```python
from build123d import *

# Parameters (mm, degrees)
BOSS_EXTRUDE1_DEPTH      = 1.7
BOSS_EXTRUDE1_DEPTH_BACK = 1.7
SKETCH1_R                = 2.7
SKETCH1_R_2              = 1.5
SKETCH1_R_3              = 3.5


with BuildPart() as part:
    # Sketch1 → Boss-Extrude1 (new, two sides: drawn at the far end of the back side and taken through both)
    # profile 1 of 3: a face of its own
    with BuildSketch(Plane(origin=(0, 0, 0), x_dir=(0, 0, -1), z_dir=(1, 0, 0)).offset(-BOSS_EXTRUDE1_DEPTH_BACK)):
        with BuildLine():
            Line((43.152237127, 13.072535054), (4.028300378, -1.651140858))
            ThreePointArc((4.028300378, -1.651140858), (6.515897328, -1.95802161), (7.67928888, -4.178119463))
            ThreePointArc((7.67928888, -4.178119463), (7.169578833, -5.756925949), (5.832896346, -6.739633526))
            Line((5.832896346, -6.739633526), (45.491528196, 6.476340855))
            ThreePointArc((45.491528196, 6.476340855), (41.086299002, 8.626962345), (43.152237127, 13.072535054))
        make_face()
    # profile 2 of 3: a face of its own
    with BuildSketch(Plane(origin=(0, 0, 0), x_dir=(0, 0, -1), z_dir=(1, 0, 0)).offset(-BOSS_EXTRUDE1_DEPTH_BACK)):
        with Locations((4.97928888, -4.178119463)):
            Circle(SKETCH1_R)
        with Locations((4.97928888, -4.178119463)):
            Circle(SKETCH1_R_2, mode=Mode.SUBTRACT)
    # profile 3 of 3: a face of its own
    with BuildSketch(Plane(origin=(0, 0, 0), x_dir=(0, 0, -1), z_dir=(1, 0, 0)).offset(-BOSS_EXTRUDE1_DEPTH_BACK)):
        with Locations((44.385, 9.796822048)):
            Circle(SKETCH1_R_3)
        with Locations((44.385, 9.796822048)):
            Circle(SKETCH1_R_2, mode=Mode.SUBTRACT)
    extrude(amount=BOSS_EXTRUDE1_DEPTH + BOSS_EXTRUDE1_DEPTH_BACK)


solid = part.part
```
Geometry check sheet. Reference: the model listing, model coordinates, mm. Give positions to 0.01 mm unless a question says otherwise; leave off trailing zeros. Loops run counter-clockwise (first coordinate to the right, second up) from the corner with the lowest first, then second, coordinate; pieces in that order, holes last. Notation, with made-up numbers: M 9.5,-33 L 38.5,-33 A19 ccw 38.5,-20 Z; hole C 61.5,66 d9. An arc over 180 degrees is marked long. Write item = value, one per line.
(1) Sectioned sample at D-D, the plane y = 2. Record the cut outline in (x, z).
Answer below:
outline = M -1.7,-32.06 L 1.7,-32.06 L 1.7,-13.73 L -1.7,-13.73 Z
(2) Material ranges on line 1 (Y direction, x = -1.05, z = -6); line 2 (Y direction, x = -0.9, z = -27.5); line 3 (Y direction, x = 1.5, z = -44), recorded low to high. Write a range as [from, to].
Answer below:
line_1 = [-6.68, -5.28], [-3.08, -0.91]
line_2 = [0.48, 7.18]
line_3 = [5.98, 8.35], [11.25, 13.28]
(3) Release check for a two-part mould opening along Z. For faces 1 (the face through (-0.02, -5.09, -3.79)), 2 (the face through (-0.024, -0.224, -25.385)), 3 (the face through (1.7, 3, -25)), 4 (the face through (-0.024, 5.814, -23.864)) record: released by +Z, released by -Z, zero draft, split by the parting line, or undercut.
Answer below:
face_1 = undercut
face_2 = released by -Z
face_3 = zero draft
face_4 = released by +Z
(4) Sectioned sample at A-A, the plane z = -44. Record the cut outline in (x, y), plus the area to 3 significant figures.
Answer below:
outline = M -1.7,5.98 L 1.7,5.98 L 1.7,8.35 L -1.7,8.35 Z; M -1.7,11.25 L 1.7,11.25 L 1.7,13.28 L -1.7,13.28 Z
area = 14.9 mm2
(5) Sectioned sample at B-B, the plane x = 1.2. Record the cut outline in (y, z) (3 decimals).
Answer below:
outline = M -6.74,-5.833 L 6.476,-45.492 A3.5 ccw long 13.073,-43.152 L -1.651,-4.028 A2.7 ccw Z; hole C -4.178,-4.979 d3; hole C 9.797,-44.385 d3
(6) Gauge pin test, flat ends, axial feed: pin 1 Ø2 at (x, z) = (-0.5, -18) entering from -Y; pin 2 Ø1 at (x, z) = (1.5, -20) entering from -Y; pin 3 Ø2 at (x, z) = (-0.5, -19.5) entering from +Y. Record the tip position at first contact, or that the pin passes through.
Answer below:
pin_1 = -3.02
pin_2 = -2.19
pin_3 = 4.55
(7) Sectioned sample at C-C, the plane z = -38. Record the cut outline in (x, y), plus the area to 3 significant figures.
Answer below:
outline = M -1.7,3.98 L 1.7,3.98 L 1.7,11.13 L -1.7,11.13 Z
area = 24.3 mm2
